Check sheet for the modelled part. Datum: model origin and axes. Units: mm. A direction names the side the tool comes from. Give positions to 0.01 mm unless a question says otherwise; leave off trailing zeros. Write each loop counter-clockwise with the first axis right and the second up, starting at its lowest first coordinate (ties: lowest second). Pieces come first, ordered by that corner, then holes. Notation, with made-up numbers: M -39,13 L 4,13 A25 cw 4,43 Z; hole C 49,-31 d11. An arc over 180 degrees is marked long. Write item = value, one per line. Start each with the question number.
1) Cross-section at D-D, the plane z = -5.5. Record the cut outline in (x, y).
2) Cross-section at C-C, the plane y = -6.25. Record the cut outline in (x, z), plus the area to 3 significant figures.
3) Access from +Z, -Z, +X, -X, +Y, -Y to the whole of each face (thin tool, end or side, straight path). Record for faces 4 (the cylindrical face through (-2.579, -0.978, -5.916)), 5 (the flat face through (-2.5, 5, -2)), 6 (the flat face through (-0.3, -6.8, -7.5)), 7 (the flat face through (0, 1, -13.5)), 8 (the flat face through (4, 3.5, -2)).
4) Mould release check, pull along X, two halves, no side actions. Record for faces 1 (the flat face through (1.75, -4, -14)), 2 (the cylindrical face through (0, -9, -13.2)), 3 (the flat face through (-3, -4, -14.5)): released by +X, released by -X, zero draft, split by the parting line, or undercut.
5) Cross-section at A-A, the plane z = -2. Record the cut outline in (x, y), plus the area to 3 significant figures.
6) Go/stop test with flat-tipped pins: pin 1 (1.5 mm diameter, centred on x = 3.5, z = -7, fed in from +Y); pin 2 (1.3 mm diameter, centred on x = 1, y = 3.5, fed in from -Z); pin 3 (4.5 mm diameter, centred on x = -1, y = 4.5, fed in from -Z). Record where each tip stops, or that it passes through.
7) Cross-section at B-B, the plane z = -7.25. Record the cut outline in (x, y), plus the area to 3 significant figures.
8) Scan lines: line 1 along Y through (x, z) = (0, -13.15); line 2 along Y through (x, z) = (-0.5, -1); line 3 along X through (y, z) = (1.75, -6.5). Record each from-to range of solid material in increasing order. Write a range as [from, to].
```python
from build123d import *

# Parameters (mm, degrees)
SKETCH1_W           = 9
SKETCH1_H           = 11
BOSS_EXTRUDE1_DEPTH = 14.5
CUT_EXTRUDE3_DEPTH  = 11
SKETCH3_W           = 3
SKETCH3_H           = 6.8
CUT_EXTRUDE4_DEPTH  = 0.3
SKETCH5_W           = 1.5
SKETCH5_H           = 7.5
CUT_EXTRUDE5_DEPTH  = 18.781732199
SKETCH6_W           = 3.5
SKETCH6_H           = 3.5
CUT_EXTRUDE6_DEPTH  = 1.5
BOSS_EXTRUDE2_DEPTH = 0.5
SKETCH8_R           = 1.375
SKETCH8_R_2         = 1
BOSS_EXTRUDE3_DEPTH = 0.5
CHAMFER1_SIZE       = 0.5
SKETCH9_W           = 2.5
SKETCH9_H           = 0.5
BOSS_EXTRUDE4_DEPTH = 6
CUT_EXTRUDE8_DEPTH  = 0.5
SKETCH11_R          = 0.6
CUT_EXTRUDE9_DEPTH  = 17.83745824
SKETCH12_W          = 1.5
SKETCH12_H          = 2
CUT_EXTRUDE10_DEPTH = 2
SKETCH13_R          = 3.25
SKETCH13_R_2        = 1
CUT_EXTRUDE11_DEPTH = 12
FILLET1_R           = 1
FILLET2_R           = 0.5


with BuildPart() as part:
    # Sketch1 → Boss-Extrude1 (new body)
    with BuildSketch(Plane.XY):
        Rectangle(SKETCH1_W, SKETCH1_H)
    extrude(amount=-BOSS_EXTRUDE1_DEPTH)

    # Sketch2 → Cut-Extrude3 (cut)
    with BuildSketch(Plane(origin=(0, 0, -14.5), x_dir=(-1, 0, 0), z_dir=(0, 0, -1))):
        with BuildLine():
            Line((-4.5, 1.3), (-4.2, 1.3))
            ThreePointArc((-4.2, 1.3), (-2.969848481, 4.269848481), (0, 5.5))
            Line((0, 5.5), (-4.5, 5.5))
            Line((-4.5, 5.5), (-4.5, 1.3))
        make_face()
        with BuildLine():
            ThreePointArc((0, 5.5), (2.969848481, 4.269848481), (4.2, 1.3))
            Line((4.2, 1.3), (4.5, 1.3))
            Line((4.5, 1.3), (4.5, 5.5))
            Line((4.5, 5.5), (0, 5.5))
        make_face()
    extrude(amount=-CUT_EXTRUDE3_DEPTH, mode=Mode.SUBTRACT)

    # Sketch3 → Cut-Extrude4 (cut)
    with BuildSketch(Plane(origin=(4.5, 0, 0), x_dir=(0, 0, -1), z_dir=(1, 0, 0))):
        with Locations((13, -2.1)):
            Rectangle(SKETCH3_W, SKETCH3_H)
    cut_extrude4 = extrude(amount=-CUT_EXTRUDE4_DEPTH, mode=Mode.SUBTRACT)

    # Mirror1: Cut-Extrude4 across plane
    add(cut_extrude4.mirror(Plane(origin=(0, 0, 0), x_dir=(0, 0, 1), z_dir=(1, 0, 0))), mode=Mode.SUBTRACT)

    # Sketch5 → Cut-Extrude5 (cut, through all)
    with BuildSketch(Plane(origin=(4.2, 0, 0), x_dir=(0, 0, -1), z_dir=(1, 0, 0))):
        with Locations((13.75, 1.75)):
            Rectangle(SKETCH5_W, SKETCH5_H)
    extrude(amount=-CUT_EXTRUDE5_DEPTH, mode=Mode.SUBTRACT)

    # Sketch6 → Cut-Extrude6 (cut)
    with BuildSketch(Plane(origin=(0, 0, -14.5), x_dir=(-1, 0, 0), z_dir=(0, 0, -1))):
        with Locations((0, -3.75)):
            Rectangle(SKETCH6_W, SKETCH6_H)
    extrude(amount=-CUT_EXTRUDE6_DEPTH, mode=Mode.SUBTRACT)

    # Sketch7 → Boss-Extrude2 (add)
    with BuildSketch(Plane(origin=(0, 0, -13), x_dir=(-1, 0, 0), z_dir=(0, 0, -1))):
        with BuildLine():
            Line((1.5, 1.3), (1.5, -7.5))
            ThreePointArc((1.5, -7.5), (0, -9), (-1.5, -7.5))
            Line((-1.5, -7.5), (-1.5, 1.3))
            ThreePointArc((-1.5, 1.3), (0, 2.8), (1.5, 1.3))
        make_face()
    extrude(amount=BOSS_EXTRUDE2_DEPTH)

    # Sketch8 → Boss-Extrude3 (add)
    with BuildSketch(Plane(origin=(0, 0, -13.5), x_dir=(-1, 0, 0), z_dir=(0, 0, -1))):
        with Locations((0, 1.3)):
            Circle(SKETCH8_R)
        with Locations((0, 1.3)):
            Circle(SKETCH8_R_2, mode=Mode.SUBTRACT)
    extrude(amount=BOSS_EXTRUDE3_DEPTH)

    # Chamfer1
    # the kernel refuses this chamfer: 0.5 mm, written as the material it takes off along each edge
    with BuildSketch(Plane(origin=(0, 1.3, -14), x_dir=(-1, 0, 0), z_dir=(0, -1, 0))) as chamfer1_piece_1_section:
        Polygon((1.375, -CHAMFER1_SIZE), (1.375 - CHAMFER1_SIZE, 0), (1.375, 0), align=None)
    chamfer1_piece_1 = revolve(axis=Axis((0, 1.3, -14), (0, 0, -1)), mode=Mode.PRIVATE)
    chamfer1_piece_1 = split(chamfer1_piece_1, bisect_by=Plane(origin=(1.125101861, 1.3, -13.5), z_dir=(0, 0, -1)), keep=Keep.TOP, mode=Mode.PRIVATE)
    add(chamfer1_piece_1, mode=Mode.SUBTRACT)

    # Sketch9 → Boss-Extrude4 (add)
    with BuildSketch(Plane.XZ.offset(5.5)):
        with Locations((0, -7.25)):
            Rectangle(SKETCH9_W, SKETCH9_H)
    extrude(amount=BOSS_EXTRUDE4_DEPTH)

    # Sketch10 → Cut-Extrude8 (cut)
    with BuildSketch(Plane.XY.offset(-7)):
        with BuildLine():
            ThreePointArc((1.25, -8.329156198), (0, -9), (-1.25, -8.329156198))
            Line((-1.25, -8.329156198), (-1.25, -11.5))
            Line((-1.25, -11.5), (1.25, -11.5))
            Line((1.25, -11.5), (1.25, -8.329156198))
        make_face()
    extrude(amount=-CUT_EXTRUDE8_DEPTH, mode=Mode.SUBTRACT)

    # Sketch11 → Cut-Extrude9 (cut, through all)
    with BuildSketch(Plane(origin=(0, 0, -13.5), x_dir=(-1, 0, 0), z_dir=(0, 0, -1))):
        with Locations((0, -7.5)):
            Circle(SKETCH11_R)
    extrude(amount=-CUT_EXTRUDE9_DEPTH, mode=Mode.SUBTRACT)

    # Sketch12 → Cut-Extrude10 (cut)
    with BuildSketch(Plane(origin=(4.5, 0, 0), x_dir=(0, 0, -1), z_dir=(1, 0, 0))):
        with Locations((1.75, 4.5)):
            Rectangle(SKETCH12_W, SKETCH12_H)
    cut_extrude10 = extrude(amount=-CUT_EXTRUDE10_DEPTH, mode=Mode.SUBTRACT)

    # Mirror2: Cut-Extrude10 across plane
    add(cut_extrude10.mirror(Plane(origin=(0, 0, 0), x_dir=(0, 0, 1), z_dir=(1, 0, 0))), mode=Mode.SUBTRACT)

    # Sketch13 → Cut-Extrude11 (cut)
    with BuildSketch(Plane.XY):
        with Locations((0, 1)):
            Circle(SKETCH13_R)
        with Locations((0, 1)):
            Circle(SKETCH13_R_2, mode=Mode.SUBTRACT)
    extrude(amount=-CUT_EXTRUDE11_DEPTH, mode=Mode.SUBTRACT)

    # Fillet1
    fillet1_edges = [part.edges().sort_by_distance(p)[0] for p in [
        (-1, 1, 0),
    ]]
    fillet(fillet1_edges, radius=FILLET1_R)

    # Fillet2
    fillet2_edges = [part.edges().sort_by_distance(p)[0] for p in [
        (4.5, 5.5, -3),
        (4.5, 5.5, -0.5),
        (-4.5, 5.5, -0.5),
        (-4.5, 5.5, -3),
        (0, -5.5, 0),
        (-4.5, 0, 0),
        (0, 5.5, 0),
        (4.5, 0, 0),
    ]]
    fillet(fillet2_edges, radius=FILLET2_R)


solid = part.part
```
Reply:
q1.outline = M -4.5,-5.5 L 4.5,-5.5 L 4.5,1.3 L 4.2,1.3 A4.2 ccw -4.2,1.3 L -4.5,1.3 Z; C 0,1 d2; hole C 0,1 d6.5
q2.outline = M -1.5,-13.5 L 1.5,-13.5 L 1.5,-13 L -1.5,-13 Z; M -1.25,-7.5 L 1.25,-7.5 L 1.25,-7 L -1.25,-7 Z
q2.area = 2.75 mm2
q3.face_4 = +Z
q3.face_5 = -X, +Y
q3.face_6 = +X, -X, -Y
q3.face_7 = -Z
q3.face_8 = +X, +Y
q4.face_1 = undercut
q4.face_2 = split by the parting line
q4.face_3 = zero draft
q5.outline = M -4.5,-5.5 L 4.5,-5.5 L 4.5,3.5 L 2.5,3.5 L 2.5,5.5 L -2.5,5.5 L -2.5,3.5 L -4.5,3.5 Z; C 0,1 d2; hole C 0,1 d6.5
q5.area = 61.0 mm2
q6.pin_1 = 4.47
q6.pin_2 = -13
q6.pin_3 = -13.77
q7.outline = M -4.5,-5.5 L -1.25,-5.5 L -1.25,-8.33 A1.5 ccw 1.25,-8.33 L 1.25,-5.5 L 4.5,-5.5 L 4.5,1.3 L 4.2,1.3 A4.2 ccw -4.2,1.3 L -4.5,1.3 Z; C 0,1 d2; hole C 0,1 d6.5; hole C 0,-7.5 d1.2
q7.area = 66.0 mm2
q8.line_1 = [-9, -8.1], [-6.9, 2.8]
q8.line_2 = [-5.5, -2.21], [0.13, 1.87], [4.21, 5.5]
q8.line_3 = [-4.18, -3.16], [-0.66, 0.66], [3.16, 4.18]
